The figure shows three views and two pictorial views of one solid part (mm, origin at its lowest corner). Answer the questions. Coordinates: 2 decimals unless noted, no trailing zeros. Loops run counter-clockwise (first coordinate to the right, second up) from the corner with the lowest first, then second, coordinate; pieces in that order, holes last. Notation, with made-up numbers: (44, 26) - (87, 26) arc R15 cw to (87, 44) - close; hole circle Ø3 at (12, 39.25). An arc over 180 degrees is marked (long way). Return JSON: item names as keys, results as strings. Group by question number.
1. Find the intervals of material crossed by line 1 along Z through (x, y) = (14, 2.15); line 2 along X through (y, z) = (0.95, 24); line 3 along Z through (x, y) = (8, 1.05), in increasing order.
2. Section A-A (x = 8.75) is taken. Write down the section's boundary in (y, z), and give its area (3 significant figures).
3. Section D-D (y = 1.4) is taken. Write down the section's boundary in (x, z).
4. Section B-B (z = 20) is taken. Write down the section's boundary in (x, y).
5. Section C-C (x = 5.5) is taken. Write down the section's boundary in (y, z), and give its area (3 significant figures).
6. This flat-tipped pin is pushed along its axis until it touches: P1, Ø2.5, axis at x = 27, z = 35, coming from the +Y side. Where does it stop, or does it pass through?
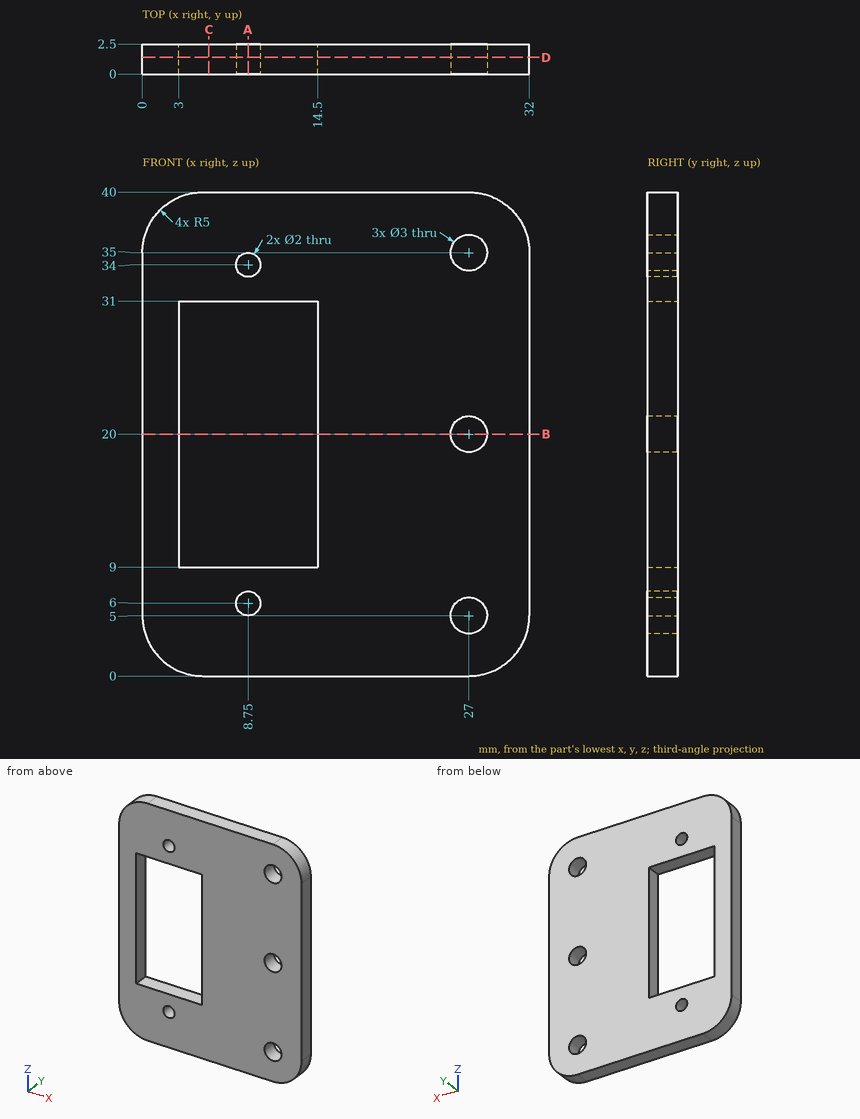
The answers:
{
 "1": {"line 1": "z = 0 to 9, 31 to 40", "line 2": "x = 0 to 3, 14.5 to 32", "line 3": "z = 0 to 5.34, 6.66 to 9, 31 to 33.34, 34.66 to 40"},
 "2": {"outline": "(0, 0) - (2.5, 0) - (2.5, 5) - (0, 5) - close; (0, 7) - (2.5, 7) - (2.5, 9) - (0, 9) - close; (0, 31) - (2.5, 31) - (2.5, 33) - (0, 33) - close; (0, 35) - (2.5, 35) - (2.5, 40) - (0, 40) - close", "area": "35.0 mm2"},
 "3": {"outline": "(0, 5) arc R5 ccw to (5, 0) - (27, 0) arc R5 ccw to (32, 5) - (32, 35) arc R5 ccw to (27, 40) - (5, 40) arc R5 ccw to (0, 35) - close; hole (3, 9) - (14.5, 9) - (14.5, 31) - (3, 31) - close; hole circle Ø2 at (8.75, 6); hole circle Ø2 at (8.75, 34); hole circle Ø3 at (27, 5); hole circle Ø3 at (27, 20); hole circle Ø3 at (27, 35)"},
 "4": {"outline": "(0, 0) - (3, 0) - (3, 2.5) - (0, 2.5) - close; (14.5, 0) - (25.5, 0) - (25.5, 2.5) - (14.5, 2.5) - close; (28.5, 0) - (32, 0) - (32, 2.5) - (28.5, 2.5) - close"},
 "5": {"outline": "(0, 0) - (2.5, 0) - (2.5, 9) - (0, 9) - close; (0, 31) - (2.5, 31) - (2.5, 40) - (0, 40) - close", "area": "45.0 mm2"},
 "6": {"P1": "passes through"}
}
